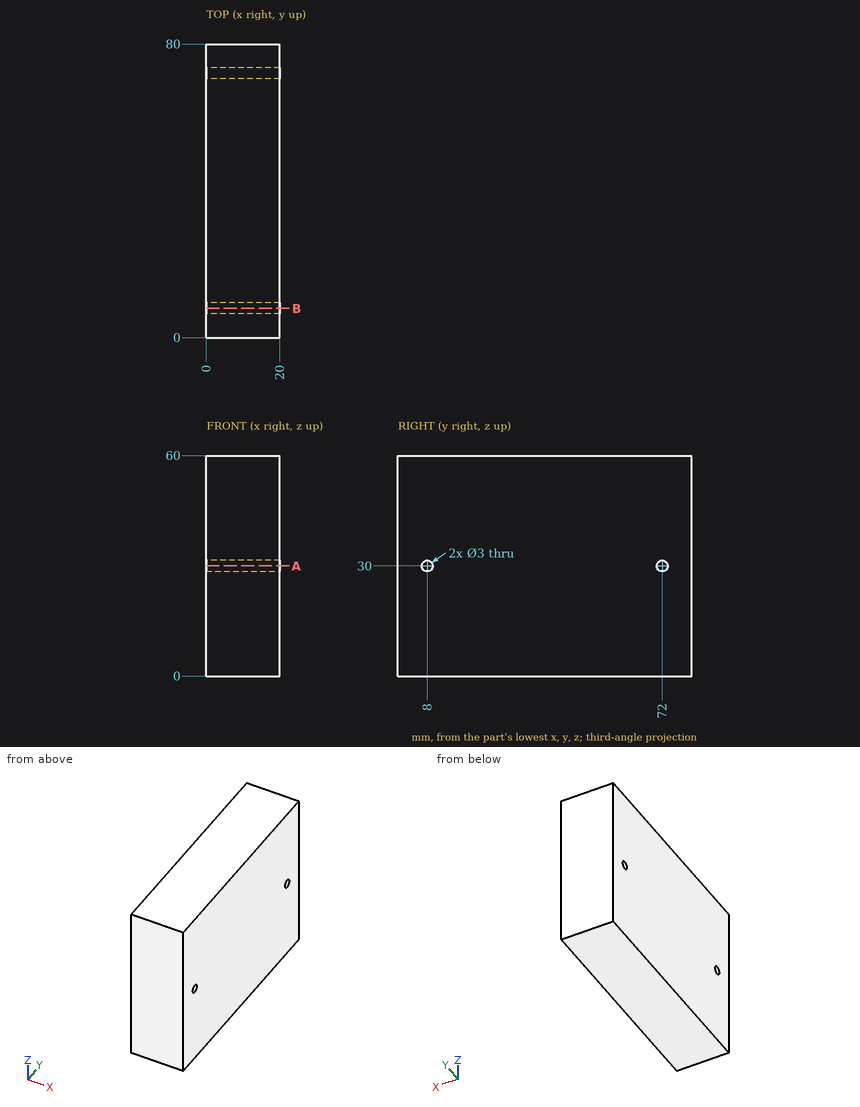
For this review, use the dimensioned drawing (mm, ordinates from the lowest corner) and the shaded views. Round coordinates to 2 decimals unless told otherwise and drop trailing zeros. Loops run counter-clockwise (first coordinate to the right, second up) from the corner with the lowest first, then second, coordinate; pieces in that order, holes last. Notation, with made-up numbers: M 36,85.5 L 65,85.5 A10 ccw 65,97.5 Z; hole C 78,63.5 d4. An arc over 180 degrees is marked long. Answer as CSV lines item,"result".
1. We need section A-A (z = 30). Give the boundary of the cut face in (x, y), plus the area to 3 significant figures.
Outcome:
outline,"M 0,0 L 20,0 L 20,6.5 L 0,6.5 Z; M 0,9.5 L 20,9.5 L 20,70.5 L 0,70.5 Z; M 0,73.5 L 20,73.5 L 20,80 L 0,80 Z"
area,"1,480 mm2"
2. To check wall thickness, follow L1, parallel to Y at x = 14.5, z = 30; L2, parallel to Z at x = 6.25, y = 8. State the ranges of each line that lie inside material, in increasing order. Write a range as [from, to].
Outcome:
L1,"y = [0, 6.5], [9.5, 70.5], [73.5, 80]"
L2,"z = [0, 28.5], [31.5, 60]"
3. We need section B-B (y = 8). Give the boundary of the cut face in (x, z).
Outcome:
outline,"M 0,0 L 20,0 L 20,28.5 L 0,28.5 Z; M 0,31.5 L 20,31.5 L 20,60 L 0,60 Z"
